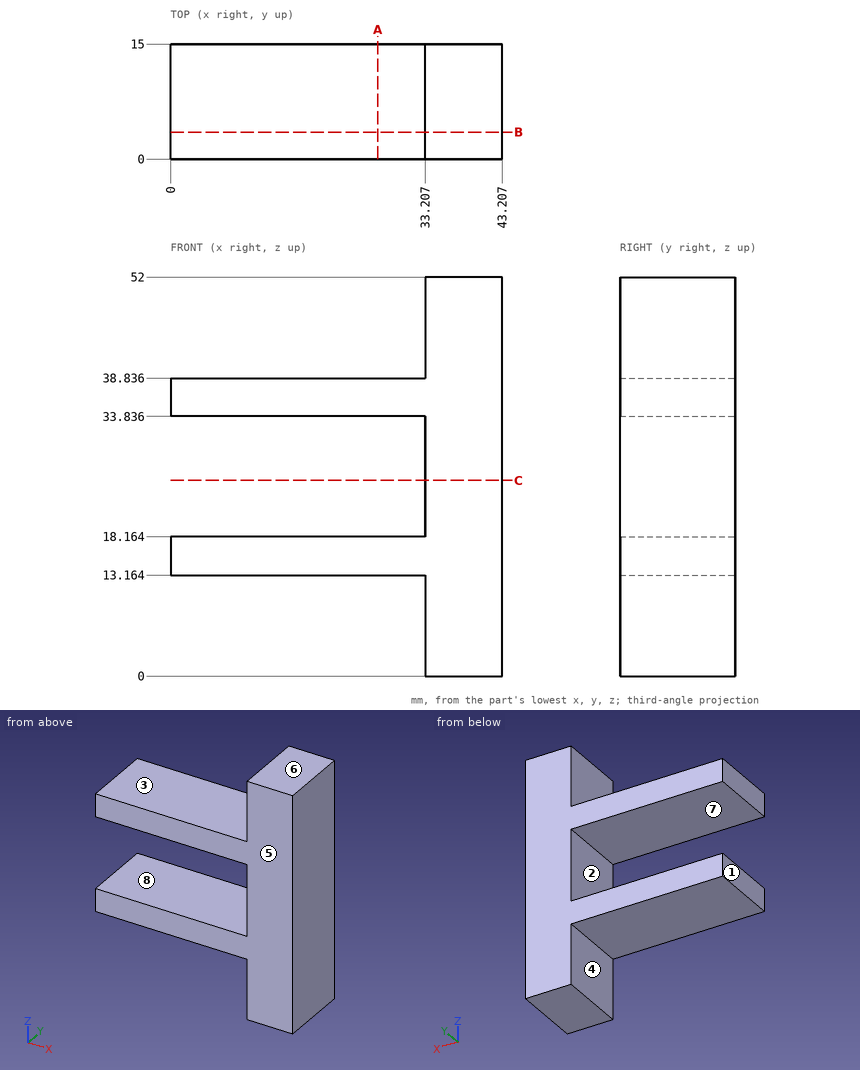
Job drawing, mm, ordinate dimensions from the low corner. One solid piece. A direction names the side the tool comes from. Give positions to 0.01 mm unless a question says otherwise; leave off trailing zeros. Loops run counter-clockwise (first coordinate to the right, second up) from the corner with the lowest first, then second, coordinate; pieces in that order, holes last.
Item 1: Pull direction Z, two halves, no side cores. Call the marked faces 5, 6, 7 and 8: released by +Z, released by -Z, zero draft, split by the parting line, or undercut.
Answers follow:
face 5: zero draft
face 6: released by +Z
face 7: undercut
face 8: undercut
Item 2: Slice it at A-A, the plane x = 27. List the corners of the cut face in (y, z), and give its area (3 significant figures).
Answers follow:
outline: (0, 13.16) - (15, 13.16) - (15, 18.16) - (0, 18.16) - close; (0, 33.84) - (15, 33.84) - (15, 38.84) - (0, 38.84) - close
area: 150 mm2
Item 3: Slice it at C-C, the plane z = 25.5. List the corners of the cut face in (x, y), and give its area (3 significant figures).
Answers follow:
outline: (33.21, 0) - (43.21, 0) - (43.21, 15) - (33.21, 15) - close
area: 150 mm2
Item 4: Which spindle directions (+Z, -Z, +X, -X, +Y, -Y) get a long thin tool onto all of the face, cutting with end or side? Do the marked faces 1, 2, 3 and 4. Say none if no direction does.
Answers follow:
face 1: +Z, -Z, -X, +Y, -Y
face 2: -X, +Y, -Y
face 3: +Z, -X, +Y, -Y
face 4: -Z, -X, +Y, -Y
Item 5: Drill centre lines: line 1 (Z direction, x = 19, y = 2.5); line 2 (X direction, y = 6.5, z = 27). Where is each one in solid material? Low to high.
Answers follow:
line 1: z = 13.16 to 18.16, 33.84 to 38.84
line 2: x = 33.21 to 43.21
Item 6: Slice it at B-B, the plane y = 3.5. List the corners of the cut face in (x, z).
Answers follow:
outline: (0, 13.16) - (33.21, 13.16) - (33.21, 0) - (43.21, 0) - (43.21, 52) - (33.21, 52) - (33.21, 38.84) - (0, 38.84) - (0, 33.84) - (33.21, 33.84) - (33.21, 18.16) - (0, 18.16) - close
Item 7: Flat gauge pins, fed straight in: pin 1 (4 mm diameter, centred on y = 7.5, z = 5, fed in from -X); pin 2 (4.5 mm diameter, centred on x = 13, y = 4.5, fed in from +Z); pin 3 (7.5 mm diameter, centred on x = 17.5, y = 11, fed in from -Z). Where does each tip first touch, or does it go through?
Answers follow:
pin 1: stops at x = 33.21
pin 2: stops at z = 38.84
pin 3: stops at z = 13.16
